```python
from build123d import *

# Parameters (mm, degrees)
F0_W     = 67.1
F0_H     = 138.3
F1_DEPTH = 15
F2_R     = 5
F3_T     = -2.5


# Not quite as in the source:
# - a shell that OpenCascade refuses in one call is made with other operations: the cavity is built on its own and cut out


with BuildPart() as f1:
    # F0 (on Front) → F1 (new body)
    with BuildSketch(Plane.XZ):
        Rectangle(F0_W, F0_H)
    extrude(amount=-F1_DEPTH)

    # F2
    f2_edges = [f1.edges().sort_by_distance(p)[0] for p in [
        (-33.55, 7.5, 69.15),
        (33.55, 7.5, 69.15),
        (-33.55, 7.5, -69.15),
        (33.55, 7.5, -69.15),
    ]]
    fillet(f2_edges, radius=F2_R)

    # F3: a shell. OpenCascade refuses it in one call, so the cavity is built on its own and cut out:
    # the body offset inwards by the wall thickness, plus a prism from it out through each open face.
    f3_core = offset(f1.part, amount=F3_T, mode=Mode.PRIVATE)
    f3_exits = [f3_core.faces().sort_by_distance(p)[0] for p in [
        (0, 7.5, 66.65),
    ]]
    add(f3_core, mode=Mode.SUBTRACT)
    extrude(f3_exits, amount=-F3_T, mode=Mode.SUBTRACT)


solid = f1.part
```
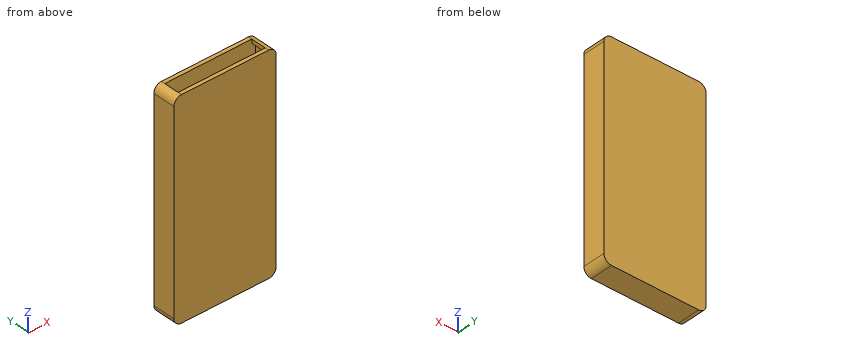
For this review, take the finished solid that the model builds, in its own axes (mm). Round coordinates to 2 decimals unless told otherwise and drop trailing zeros. Loops run counter-clockwise (first coordinate to the right, second up) from the corner with the lowest first, then second, coordinate; pieces in that order, holes last.
(1) Wall thickness on line 1 along Y through (x, z) = (-0.5, 38); line 2 along X through (y, z) = (9.25, 39.5); line 3 along Z through (x, y) = (-17, 4.25): over which ranges is each line inside the solid? List them lowest first.
Returned:
line 1: y = 0 to 2.5, 12.5 to 15
line 2: x = -33.55 to -31.05, 31.05 to 33.55
line 3: z = -69.15 to -66.65
(2) We need section B-B (z = 52). Give the boundary of the cut face in (x, y).
Returned:
outline: (-33.55, 0) - (33.55, 0) - (33.55, 15) - (-33.55, 15) - close; hole (-31.05, 2.5) - (31.05, 2.5) - (31.05, 12.5) - (-31.05, 12.5) - close
(3) We need section C-C (y = 6.5). Give the boundary of the cut face in (x, z).
Returned:
outline: (-33.55, -64.15) arc R5 ccw to (-28.55, -69.15) - (28.55, -69.15) arc R5 ccw to (33.55, -64.15) - (33.55, 64.15) arc R5 ccw to (28.55, 69.15) - (28.55, 66.65) arc R2.5 cw to (31.05, 64.15) - (31.05, -64.15) arc R2.5 cw to (28.55, -66.65) - (-28.55, -66.65) arc R2.5 cw to (-31.05, -64.15) - (-31.05, 64.15) arc R2.5 cw to (-28.55, 66.65) - (-28.55, 69.15) arc R5 ccw to (-33.55, 64.15) - close
(4) We need section A-A (x = 0). Give the boundary of the cut face in (y, z).
Returned:
outline: (0, -69.15) - (15, -69.15) - (15, 69.15) - (12.5, 69.15) - (12.5, -66.65) - (2.5, -66.65) - (2.5, 69.15) - (0, 69.15) - close
(5) Clearance check with flat-ended pins moving along their axes: P1, Ø1.2, axis at y = 6.5, z = 68, coming from the -X side; P2, Ø3, axis at x = 23.5, y = 7.5, coming from the +Z side; P3, Ø3, axis at y = 6.5, z = 68, coming from the +X side. State where each tip first meets the part, or that it passes through.
Returned:
P1: stops at x = -32.35
P2: stops at z = -66.65
P3: stops at x = 32.96
